```python
from build123d import *

# Parameters (mm, degrees)
SKETCH1_W           = 60
SKETCH1_H           = 30
BOSS_EXTRUDE1_DEPTH = 10
SKETCH2_W           = 41
SKETCH2_H           = 20
CUT_EXTRUDE1_DEPTH  = 10
SKETCH3_R           = 1.5
SKETCH3_W           = 14
SKETCH3_H           = 1.2
CUT_EXTRUDE2_DEPTH  = 4
FILLET1_R           = 2
CHAMFER1_SIZE       = 2
SKETCH5_W           = 145.508726569
SKETCH5_H           = 79.029504781
CUT_EXTRUDE3_DEPTH  = 4


with BuildPart() as part:
    # Sketch1 → Boss-Extrude1 (new body)
    with BuildSketch(Plane.XY):
        Rectangle(SKETCH1_W, SKETCH1_H)
    extrude(amount=BOSS_EXTRUDE1_DEPTH)

    # Sketch2 → Cut-Extrude1 (cut)
    with BuildSketch(Plane.XY.offset(10)):
        Rectangle(SKETCH2_W, SKETCH2_H)
    extrude(amount=-CUT_EXTRUDE1_DEPTH, mode=Mode.SUBTRACT)

    # Sketch3 → Cut-Extrude2 (cut)
    with BuildSketch(Plane.XY.offset(10)):
        with Locations((-24.5, 4.75)):
            Circle(SKETCH3_R)
        with Locations(Location((-24.5, -4.75, 0), (0, 0, 180))):
            Circle(SKETCH3_R)
        with Locations((24.5, -4.75)):
            Circle(SKETCH3_R)
        with Locations(Location((24.5, 4.75, 0), (0, 0, 180))):
            Circle(SKETCH3_R)
        with Locations((-20.5, 0)):
            Rectangle(SKETCH3_W, SKETCH3_H)
        with Locations((20.5, 0)):
            Rectangle(SKETCH3_W, SKETCH3_H)
    extrude(amount=-CUT_EXTRUDE2_DEPTH, mode=Mode.SUBTRACT)

    # Fillet1
    fillet1_edges = [part.edges().sort_by_distance(p)[0] for p in [
        (30, -15, 5),
        (-30, -15, 5),
        (-30, 15, 5),
        (30, 15, 5),
    ]]
    fillet(fillet1_edges, radius=FILLET1_R)

    # Chamfer1
    chamfer1_edges = [part.edges().sort_by_distance(p)[0] for p in [
        (0, 15, 10),
        (30, 0, 10),
        (-30, 0, 10),
        (0, -15, 10),
        (-29.414213562, 14.414213562, 10),
        (-29.414213562, -14.414213562, 10),
        (29.414213562, -14.414213562, 10),
        (29.414213562, 14.414213562, 10),
    ]]
    chamfer(chamfer1_edges, length=CHAMFER1_SIZE - 0.0001)  # a hair under: the kernel refuses the full size

    # Sketch5 → Cut-Extrude3 (cut)
    with BuildSketch(Plane(origin=(0, 0, 0), x_dir=(-1, 0, 0), z_dir=(0, 0, -1))):
        with Locations((-37.961499545, 20.658262846)):
            Rectangle(SKETCH5_W, SKETCH5_H)
    extrude(amount=-CUT_EXTRUDE3_DEPTH, mode=Mode.SUBTRACT)


solid = part.part
```
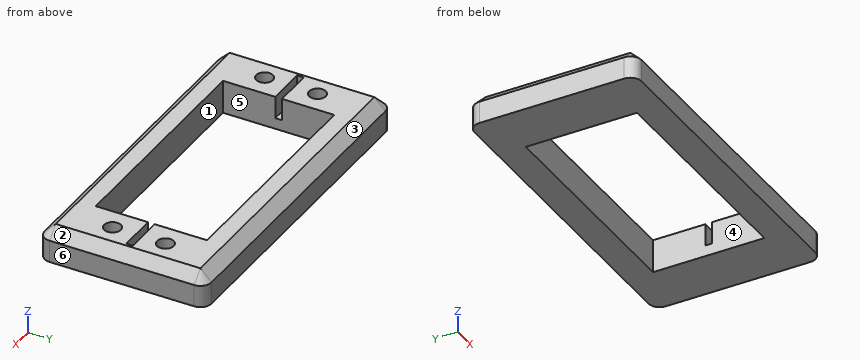
Can you work these out from the model? Positions are in its coordinate system, mm. Face numbers are marked on the shaded views. A direction names the side the tool comes from. Coordinates: 2 decimals unless noted, no trailing zeros. Loops run counter-clockwise (first coordinate to the right, second up) from the corner with the lowest first, then second, coordinate; pieces in that order, holes last. Notation, with made-up numbers: (53.25, 11.5) -> (84.25, 11.5) arc R21 ccw to (84.25, 33.5) -> close; hole circle Ø9 at (-10.5, -4.75). An arc over 180 degrees is marked (long way). Answer as a JSON object with one key per item and string values.
1) Imagine slicing it at C-C (y = -7). Please give me the cut outline in (x, z).
Results:
{"outline": "(-30, 4) -> (-20.5, 4) -> (-20.5, 10) -> (-28, 10) -> (-30, 8) -> close; (20.5, 4) -> (30, 4) -> (30, 8) -> (28, 10) -> (20.5, 10) -> close"}
2) For P1, Ø2.5, axis at x = -24.5, y = 4.75, coming from the +Z side; P2, Ø1.3, axis at x = -23.5, y = 0, coming from the +Z side; P3, Ø12, axis at x = 6, y = 0, coming from the +Z side, each with a flat end and sliding along its axis, tell me the tip position at first contact or that it passes through.
Results:
{"P1": "stops at z = 6", "P2": "stops at z = 10", "P3": "passes through"}
3) If I drill on line 1 (Y direction, x = 24.5, z = 7.55); line 2 (X direction, y = -2.5, z = 5.4); line 3 (Y direction, x = 8.5, z = 7.7), over which ranges is the centre line in solid material (lowest first)?
Results:
{"line 1": "y = -15 to -6.25, -3.25 to -0.6, 0.6 to 3.25, 6.25 to 15", "line 2": "x = -30 to -20.5, 20.5 to 30", "line 3": "y = -15 to -10, 10 to 15"}
4) For the marked faces 5 and 6, which set-ups out of +Z, -Z, +X, -X, +Y, -Y let a thin tool reach every point of the face, with its end or its side?
Results:
{"face 5": "+Z, -Z", "face 6": "+Z, -Z, +X, +Y, -Y"}
5) Imagine slicing it at D-D (z = 8.7). Please give me the cut outline in (x, y), then the cut area to 3 significant figures.
Results:
{"outline": "(-29.3, -13) arc R1.3 ccw to (-28, -14.3) -> (28, -14.3) arc R1.3 ccw to (29.3, -13) -> (29.3, 13) arc R1.3 ccw to (28, 14.3) -> (-28, 14.3) arc R1.3 ccw to (-29.3, 13) -> close; hole (-27.5, -0.6) -> (-20.5, -0.6) -> (-20.5, -10) -> (20.5, -10) -> (20.5, -0.6) -> (27.5, -0.6) -> (27.5, 0.6) -> (20.5, 0.6) -> (20.5, 10) -> (-20.5, 10) -> (-20.5, 0.6) -> (-27.5, 0.6) -> close; hole circle Ø3 at (-24.5, -4.75); hole circle Ø3 at (-24.5, 4.75); hole circle Ø3 at (24.5, -4.75); hole circle Ø3 at (24.5, 4.75)", "area": "809 mm^2"}
6) Thinking about a two-plate mould opening in Y: for the marked faces 1, 2, 3 and 4, which applies, pulls with the +Y half, pulls with the -Y half, needs draft (parallel to the pull), parting line crosses it, or undercut?
Results:
{"face 1": "undercut", "face 2": "needs draft", "face 3": "pulls with the +Y half", "face 4": "undercut"}
7) Imagine slicing it at B-B (z = 4.55). Please give me the cut outline in (x, y), then the cut area to 3 significant figures.
Results:
{"outline": "(-30, -13) arc R2 ccw to (-28, -15) -> (28, -15) arc R2 ccw to (30, -13) -> (30, 13) arc R2 ccw to (28, 15) -> (-28, 15) arc R2 ccw to (-30, 13) -> close; hole (-20.5, -10) -> (20.5, -10) -> (20.5, 10) -> (-20.5, 10) -> close", "area": "977 mm^2"}
8) Imagine slicing it at A-A (x = -10.5). Please give me the cut outline in (y, z), then the cut area to 3 significant figures.
Results:
{"outline": "(-15, 4) -> (-10, 4) -> (-10, 10) -> (-13, 10) -> (-15, 8) -> close; (10, 4) -> (15, 4) -> (15, 8) -> (13, 10) -> (10, 10) -> close", "area": "56.0 mm^2"}
